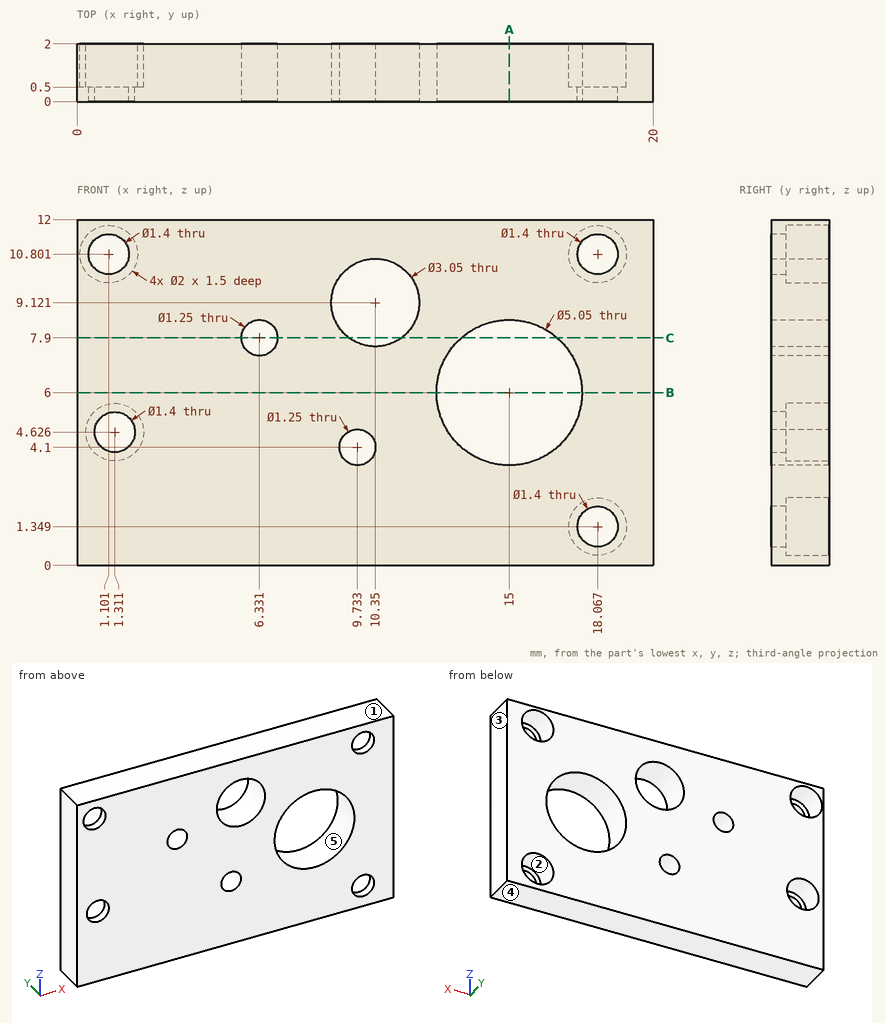
Input: dimensioned drawing with shaded views. Units: mm. Origin: part minimum x, y, z. A direction names the side the tool comes from. Coordinates: 2 decimals unless noted, no trailing zeros. Loops run counter-clockwise (first coordinate to the right, second up) from the corner with the lowest first, then second, coordinate; pieces in that order, holes last.
Q1. Section B-B, the plane z = 6. Return the cut outline in (x, y) (1 decimal).
Results are:
outline: (0, 0) - (12.5, 0) - (12.5, 2) - (0, 2) - close; (17.5, 0) - (20, 0) - (20, 2) - (17.5, 2) - close
Q2. Contact query for a flat-ended pin moving along its axis: pin 1 (1.6 mm diameter, centred on x = 18.07, z = 10.8, fed in from +Y). Output: stop coordinate, or through.
Results are:
pin 1: stops at y = 0.5
Q3. Section A-A, the plane x = 15. Return the cut outline in (y, z) (1 decimal).
Results are:
outline: (0, 0) - (2, 0) - (2, 3.5) - (0, 3.5) - close; (0, 8.5) - (2, 8.5) - (2, 12) - (0, 12) - close
Q4. Line query: line 1 along X through (y, z) = (0.3, 5); line 2 along X through (y, z) = (1.1, 9); line 3 along X through (y, z) = (1.55, 7.75) (1 decimal). Output: solid intervals per line, ascending.
Results are:
line 1: x = 0 to 0.72, 1.9 to 12.68, 17.32 to 20
line 2: x = 0 to 8.83, 11.87 to 20
line 3: x = 0 to 5.7, 6.9 to 9.7, 11 to 13.2, 16.8 to 20
Q5. Mould query, pull axis Z, two halves, no side actions, for the marked faces 3, 4 and 5. Classes: +Z half, -Z half, draft (parallel to the pull), parting line (faces both ways), or undercut.
Results are:
face 3: draft
face 4: -Z half
face 5: undercut
Q6. Section C-C, the plane z = 7.9. Return the cut outline in (x, y) (1 decimal).
Results are:
outline: (0, 0) - (5.7, 0) - (5.7, 2) - (0, 2) - close; (7, 0) - (9.4, 0) - (9.4, 2) - (7, 2) - close; (11.3, 0) - (13.3, 0) - (13.3, 2) - (11.3, 2) - close; (16.7, 0) - (20, 0) - (20, 2) - (16.7, 2) - close
Q7. Set-up query: the marked faces 1 and 2. Return all of +Z, -Z, +X, -X, +Y, -Y with unobstructed straight access to the full face (end or side cutting, diameter ignored); none if empty.
Results are:
face 1: +Z, +X, -X, +Y, -Y
face 2: +Y
